Input: part model. Units: mm. Frame: model coordinates. Round coordinates to 2 decimals unless told otherwise and drop trailing zeros. Order: outer loops, then holes, each group sorted by start corner. A loop starts at its lowest first (then second) coordinate and runs counter-clockwise, first axis right, second up. Notation, with made-up numbers: (84, 59.25) -> (121, 59.25) arc R30 cw to (121, 83.25) -> close; hole circle Ø5 at (25.25, 48). An arc over 180 degrees is marked (long way). Answer as CSV lines item,"result". Start each with the question number.
1) Line query: L1, parallel to X at y = -3.25, z = 0.75; L2, parallel to X at y = 1.5, z = 0.2; L3, parallel to Y at x = 31.75, z = 0.85. Output: solid intervals per line, ascending.
2) Section query C-C, the plane x = 13. Output: boundary loops of the cut face in (y, z).
3) Section query B-B, the plane z = 1.55. Output: boundary loops of the cut face in (x, y), and give its area (3 significant figures).
4) First-contact query: P1, Ø1, axis at y = -2.5, z = 1, coming from the +X side; P2, Ø3, axis at x = 31, y = 0.5, coming from the -Z side. Flat tips, straight axial feed; report the tip coordinate or a pass-through.
5) Section query D-D, the plane z = 0.25. Output: boundary loops of the cut face in (x, y), and give its area (3 significant figures).
```python
from build123d import *

# Parameters (mm, degrees)
SKETCH1_R           = 3
BOSS_EXTRUDE1_DEPTH = 2
CHAMFER1_SIZE       = 2


with BuildPart() as part:
    # Sketch1 → Boss-Extrude1 (new body)
    with BuildSketch(Plane.XY):
        with BuildLine():
            Line((34, -5), (15.5, -5))
            ThreePointArc((15.5, -5), (10.5, 0), (15.5, 5))
            Line((15.5, 5), (34, 5))
            ThreePointArc((34, 5), (39, 0), (34, -5))
        make_face()
        with Locations((34, 0)):
            Circle(SKETCH1_R, mode=Mode.SUBTRACT)
    extrude(amount=BOSS_EXTRUDE1_DEPTH)

    # Chamfer1
    chamfer1_edges = [part.edges().sort_by_distance(p)[0] for p in [
        (31, 0, 0),
    ]]
    chamfer(chamfer1_edges, length=CHAMFER1_SIZE - 0.0001)  # a hair under: the kernel refuses the full size


solid = part.part
```
Findings:
1,L1,"x = 11.7 to 31.26, 36.74 to 37.8"
1,L2,"x = 10.73 to 29.44, 38.56 to 38.77"
1,L3,"y = -5 to -3.49, 3.49 to 5"
2,outline,"(-4.33, 0) -> (4.33, 0) -> (4.33, 2) -> (-4.33, 2) -> close"
3,outline,"(15.5, -5) -> (34, -5) arc R5 ccw to (34, 5) -> (15.5, 5) arc R5 ccw to start; hole circle Ø6.9 at (34, 0)"
3,area,"226 mm^2"
4,P1,"stops at x = 38.58"
4,P2,"stops at z = 0.46"
5,outline,"(15.5, -5) -> (34, -5) arc R5 ccw to (34, 5) -> (15.5, 5) arc R5 ccw to start; hole circle Ø9.5 at (34, 0)"
5,area,"193 mm^2"
